Verification items for the finished model (mm, model axes). Face numbers are marked on the shaded views. A direction names the side the tool comes from. Round coordinates to 2 decimals unless told otherwise and drop trailing zeros. Write each loop counter-clockwise with the first axis right and the second up, starting at its lowest first coordinate (ties: lowest second). Pieces come first, ordered by that corner, then holes. Notation, with made-up numbers: (-26, 47) -> (-4, 47) arc R20 ccw to (-4, 59) -> close; hole circle Ø7 at (-30, 76.25). An arc over 180 degrees is marked (long way). Use CSV: the item, a comma, the result in double quotes.
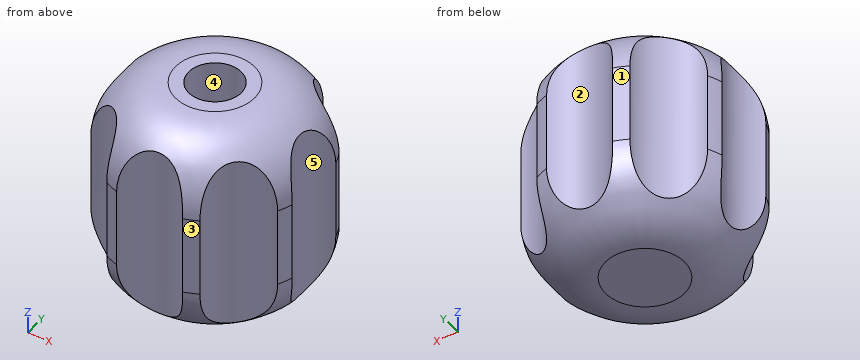
```python
from build123d import *

# Parameters (mm, degrees)
F2_R     = 5
F3_R     = 3.5
F4_DEPTH = 25


# Not quite as in the source:
# - a feature names something its author has since deleted; it is built from what else it names


with BuildPart() as f1:
    # F0 (on Front) → F1 (revolve)
    with BuildSketch(Plane.XZ):
        Polygon((-2, 4), (-2, 16), (-8, 16), (-8, 6), (-8, 0), (0, 0), (0, 4), align=None)
    revolve(axis=Axis((0, 0, 2), (0, 0, -1)))

    # F2
    f2_edges = [f1.edges().sort_by_distance(p)[0] for p in [
        (8, 0, 0),
        (8, 0, 16),
    ]]
    fillet(f2_edges, radius=F2_R)

    # F3 (on face) → F4 (cut)
    with BuildSketch(Plane(origin=(0, 0, 0), x_dir=(1, 0, 0), z_dir=(0, 0, -1))):
        with Locations((0, 10)):
            Circle(F3_R)
        with Locations((7.0710678119, 7.0710678119)):
            Circle(F3_R)
        with Locations((10, 0)):
            Circle(F3_R)
        with Locations((7.0710678119, -7.0710678119)):
            Circle(F3_R)
        with Locations((0, -10)):
            Circle(F3_R)
        with Locations((-7.0710678119, -7.0710678119)):
            Circle(F3_R)
        with Locations((-10, 0)):
            Circle(F3_R)
        with Locations((-7.0710678119, 7.0710678119)):
            Circle(F3_R)
    extrude(amount=-F4_DEPTH, mode=Mode.SUBTRACT)


solid = f1.part
```
Q1. Section check A-A (z = 8). Record the cut outline in (x, y).
Filled in:
outline,"(-7.59, -2.54) arc R8 ccw to (-7.16, -3.57) arc R3.5 cw to (-3.57, -7.16) arc R8 ccw to (-2.54, -7.59) arc R3.5 cw to (2.54, -7.59) arc R8 ccw to (3.57, -7.16) arc R3.5 cw to (7.16, -3.57) arc R8 ccw to (7.59, -2.54) arc R3.5 cw to (7.59, 2.54) arc R8 ccw to (7.16, 3.57) arc R3.5 cw to (3.57, 7.16) arc R8 ccw to (2.54, 7.59) arc R3.5 cw to (-2.54, 7.59) arc R8 ccw to (-3.57, 7.16) arc R3.5 cw to (-7.16, 3.57) arc R8 ccw to (-7.59, 2.54) arc R3.5 cw to start; hole circle Ø4 at (0, 0)"
Q2. Access from +Z, -Z, +X, -X, +Y, -Y to the whole of each face (thin tool, end or side, straight path). Record for the marked faces 4 and 5.
Filled in:
face 4,"+Z"
face 5,"+Z, -Z, +X"
Q3. Material ranges on L1, parallel to Y at x = 0, z = 9; L2, parallel to X at y = -1, z = 12.75; L3, parallel to X at y = -3.75, z = 14.75, recorded low to high.
Filled in:
L1,"-6.5 to -2, 2 to 6.5"
L2,"-6.65 to -1.73, 1.73 to 6.65"
L3,"-5.07 to 5.07"
Q4. Mould release check, pull along X, two halves, no side actions. Record for the marked faces 1, 2 and 3: released by +X, released by -X, zero draft, split by the parting line, or undercut.
Filled in:
face 1,"released by -X"
face 2,"undercut"
face 3,"released by +X"
Q5. Go/stop test with flat-tipped pins: P1, Ø4, axis at x = 6, y = -5.5, coming from the +Z side; P2, Ø3, axis at x = -3.5, z = 5.5, coming from the -Y side; P3, Ø1, axis at x = 4.5, z = 8.5, coming from the -Y side; P4, Ø3, axis at x = -4, y = -6, coming from the -Z side. Record where each tip stops, or that it passes through.
Filled in:
P1,"z = 14.89"
P2,"y = -7.59"
P3,"y = -5.39"
P4,"z = 0.8"
